For this review, take the finished solid that the model builds, in its own axes (mm). A direction names the side the tool comes from. Round coordinates to 2 decimals unless told otherwise and drop trailing zeros. Loops run counter-clockwise (first coordinate to the right, second up) from the corner with the lowest first, then second, coordinate; pieces in that order, holes last. Notation, with made-up numbers: M -2.75,23 L 21.25,23 A27 cw 21.25,60 Z; hole C -38.75,-9.5 d9. An arc over 180 degrees is marked long. Write item = value, one per line. Start each with the question number.
```python
from build123d import *

# Parameters (mm, degrees)
SKETCH_W        = 20
SKETCH_H        = 60
SKETCH_R        = 1.5
PAD_DEPTH       = 30
SKETCH001_W     = 20
SKETCH001_H     = 10
POCKET_DEPTH    = 25
SKETCH002_R     = 3
POCKET001_DEPTH = 15
CHAMFER_SIZE    = 2
CHAMFER001_SIZE = 2


with BuildPart() as part:
    # Sketch → Pad (new body)
    with BuildSketch(Plane.XY):
        with Locations((10, 30)):
            Rectangle(SKETCH_W, SKETCH_H)
        with Locations((10, 55)):
            Circle(SKETCH_R, mode=Mode.SUBTRACT)
        with Locations((10, 5)):
            Circle(SKETCH_R, mode=Mode.SUBTRACT)
    extrude(amount=PAD_DEPTH)

    # Sketch001 (on Face7 of Pad) → Pocket (cut)
    with BuildSketch(Plane(origin=(0, 0, 0), x_dir=(1, 0, 0), z_dir=(0, 0, -1))):
        with Locations((10, -5)):
            Rectangle(SKETCH001_W, SKETCH001_H)
        with Locations((10, -55)):
            Rectangle(SKETCH001_W, SKETCH001_H)
    extrude(amount=-POCKET_DEPTH, mode=Mode.SUBTRACT)

    # Sketch002 (on Face3 of Pocket) → Pocket001 (cut)
    with BuildSketch(Plane.YZ.offset(20)):
        Polygon((10, 7.8), (10, 4.8), (50, 4.8), (50, 7.8), (43.75, 7.8), (38, 14.8), (22, 14.8), (16.25, 7.8), align=None)
        with Locations((25, 9.8)):
            Circle(SKETCH002_R, mode=Mode.SUBTRACT)
        with Locations((35, 9.8)):
            Circle(SKETCH002_R, mode=Mode.SUBTRACT)
    extrude(amount=-POCKET001_DEPTH, mode=Mode.SUBTRACT)

    # Chamfer
    chamfer_edges = [part.edges().sort_by_distance(p)[0] for p in [
        (10, 0, 25),
        (10, 60, 25),
    ]]
    chamfer(chamfer_edges, length=CHAMFER_SIZE)

    # Chamfer001
    chamfer001_edges = [part.edges().sort_by_distance(p)[0] for p in [
        (10, 10, 0),
        (10, 50, 0),
    ]]
    chamfer(chamfer001_edges, length=CHAMFER001_SIZE)


solid = part.part
```
(1) Add section C-C on y = 25. Write out the cut boundary in (x, z), and give its area (3 significant figures).
(2) Add section B-B on x = 18.5. Write out the cut boundary in (y, z).
(3) Wall thickness on L1, parallel to Y at x = 10, z = 27.5; L2, parallel to X at y = 5, z = 26.6; L3, parallel to Z at x = 18, y = 14: over which ranges is each line inside the solid? List them lowest first.
(4) Tool access review of faces 1 (the flat face through (13, 47, 7.8)), 2 (the cylindrical face through (12.6, 32, 9.9)), 3 (the flat face through (13, 13, 7.8)), 4 (the flat face through (10, 10, 13)): name each direction out of +Z, -Z, +X, -X, +Y, -Y from which nothing blocks a thin tool from reaching the whole face with its end or side.
(5) Add section A-A on y = 55. Write out the cut boundary in (x, z).
(6) Draft analysis for pull direction X (two halves, no side actions). For faces 5 (the flat face through (12.605, 40.915, 11.251)), 6 (the flat face through (20, 30, 21)), 7 (the cylindrical face through (8.5, 5.07, 27.46)), state which applies: +X half, -X half, draft (parallel to the pull), parting line (faces both ways), or undercut.
(7) For pin 1 Ø2.5 at (x, y) = (12, 52) entering from -Z; pin 2 Ø6 at (x, z) = (8, 6) entering from -Y, all flat-tipped, find the tip position at first contact; note any pin that passes through.
(8) Add section D-D on x = 10.5. Count the separate pieces of the cut face and the enclosed holes in it, and give its area (3 significant figures).
Answer sheet:
q1.outline = M 0,0 L 20,0 L 20,4.8 L 5,4.8 L 5,6.8 L 20,6.8 L 20,12.8 L 5,12.8 L 5,14.8 L 20,14.8 L 20,30 L 0,30 Z
q1.area = 540 mm²
q2.outline = M 0,27 L 2,25 L 10,25 L 10,7.8 L 16.25,7.8 L 22,14.8 L 38,14.8 L 43.75,7.8 L 50,7.8 L 50,25 L 58,25 L 60,27 L 60,30 L 0,30 Z; M 10,2 L 12,0 L 48,0 L 50,2 L 50,4.8 L 10,4.8 Z; C 25,9.8 d6; C 35,9.8 d6
q3.L1 = 0 to 3.5, 6.5 to 53.5, 56.5 to 60
q3.L2 = 0 to 8.5, 11.5 to 20
q3.L3 = 0 to 4.8, 7.8 to 30
q4.face_1 = +X, +Y
q4.face_2 = +X
q4.face_3 = +X, -Y
q4.face_4 = -Z, +X, -X, -Y
q5.outline = M 0,25 L 8.5,25 L 8.5,30 L 0,30 Z; M 11.5,25 L 20,25 L 20,30 L 11.5,30 Z
q6.face_5 = draft
q6.face_6 = +X half
q6.face_7 = undercut
q7.pin_1 = 25
q7.pin_2 = 10
q8.separate_pieces = 6
q8.enclosed_holes = 0
q8.area = 1,050 mm²
